Design review of the part built by this model. Coordinates are the model's own, in mm. Face numbers are marked on the shaded views. A direction names the side the tool comes from. Coordinates: 2 decimals unless noted, no trailing zeros. Write each loop counter-clockwise with the first axis right and the second up, starting at its lowest first coordinate (ties: lowest second). Pieces come first, ordered by that corner, then holes. Notation, with made-up numbers: (-13, 63) - (42, 63) arc R17 cw to (42, 81) - close; hole circle Ø11 at (76.5, 46). An arc over 180 degrees is marked (long way). One line per item, written item: value.
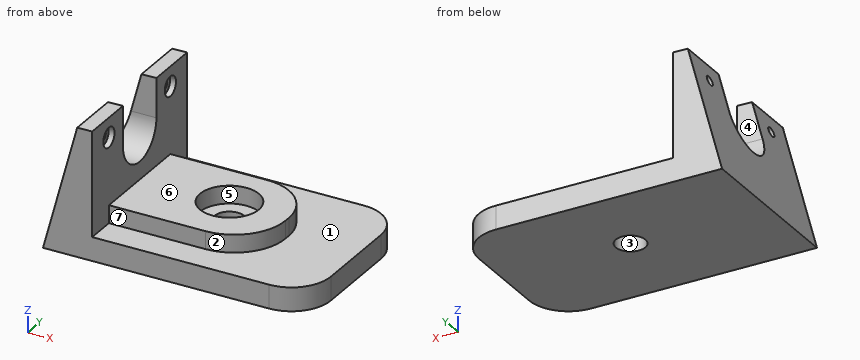
Autodesk Fusion 360 part; units mm, degrees
sketch "Baza" plane through (0, 0, 0) normal (0, 0, 1) x (1, 0, 0)
  line L0 (0, 0) -> (0, 85)
  line L1 (0, 85) -> (135, 85)
  line L2 (135, 85) -> (135, 0)
  line L3 (135, 0) -> (0, 0)
  line L4 (0, 0) -> (25, 0) construction
  line L5 (25, 0) -> (25, 85)
  line L6 (25, 85) -> (25, 70) construction
  line L7 (25, 0) -> (25, 15) construction
  line L8 (69.701, 85) -> (69.701, 0) construction
  line L9 (135, 85) -> (69.701, 44.195) construction
  circle A0 centre (69.701, 44.195) radius 7.5
  circle A1 centre (69.701, 44.195) radius 15
  line L10 (25, 70) -> (100, 70)
  line L11 (100, 70) -> (100, 15)
  line L12 (100, 15) -> (25, 15)
  line L13 (25, 15) -> (25, 70)
  dimension "d1" = 85
  dimension "d2" = 135
  dimension "d3" = 25
  dimension "d4" = 15
  dimension "d5" = 15
  dimension "d6" = 77
  dimension "d7" = 15
  dimension "d8" = 30
  dimension "d9" = 55
  dimension "d10" = 44.701
  dimension "d11" = 35
extrude "Extrude1" add sketch "Baza" along normal blind 12 contours L0 L1 L3 L5 L13 | L1 L2 L3 L5 L10 L11 L12 | L5 L10 L11 L12 L13 | A0 | A1 makes body 1
extrude "Extrude2" add sketch "Baza" along normal blind 21 separate body contours L5 L10 L11 L12 L13 makes body 2
combine "Combine1" operation add target body 2 tool bodies 1
extrude "Extrude3" cut sketch "Baza" along normal blind 50 contours A0 bodies 2
fillet "Fillet1" radius 26 2 edges at (100, 15, 16.5) (100, 70, 16.5) on bodies 2
fillet "Fillet2" radius 20 2 edges at (135, 0, 6) (135, 85, 6) on bodies 2
sketch "Margine" plane through (0, 0, 0) normal (0, -1, 0) x (1, 0, 0)
  line L0 (115, 0) -> (115, 12)
  line L1 (115, 12) -> (0, 12)
  line L2 (0, 12) -> (0, 0)
  line L3 (0, 0) -> (115, 0)
  line L4 (0, 0) -> (25, 0) construction
  line L5 (25, 0) -> (25, 65)
  line L6 (0, 0) -> (17.3848, 64.881)
  line L7 (0, 0) -> (67.1698, 0) construction
  line L8 (17.3848, 64.881) -> (25, 65)
  line L9 (3.2154, 12) -> (25, 12)
  line L10 (3.2154, 12) -> (0, 12)
  line L11 (0, 0) -> (0, 12)
  dimension "d22" = 25
  dimension "d23" = 65
  dimension "d24" = 75
extrude "Extrude4" add sketch "Margine" against normal blind 85 contours L1 L5 L6 L8 L9 bodies 2
extrude "Extrude5" cut sketch "Margine" against normal blind 85 contours L1 L2 L6 L10 L11 bodies 2
sketch "Fata" plane through (25, 0, 0) normal (1, 0, 0) x (0, 1, 0)
  line L0 (70, 21) -> (70, 12)
  line L1 (70, 12) -> (85, 12)
  line L2 (85, 12) -> (85, 65)
  line L3 (85, 65) -> (0, 65)
  line L4 (0, 65) -> (0, 12)
  line L5 (0, 12) -> (15, 12)
  line L6 (15, 12) -> (15, 21)
  line L7 (15, 21) -> (70, 21)
  line L8 (0, 65) -> (15, 65) construction
  line L9 (85, 65) -> (70, 65) construction
  line L10 (15, 65) -> (15, 55) construction
  line L11 (70, 65) -> (70, 55) construction
  circle A0 centre (15, 55) radius 2.5
  circle A1 centre (70, 55) radius 2.5
  circle A2 centre (15, 55) radius 5
  circle A3 centre (70, 55) radius 5
  line L12 (0, 65) -> (0, 45) construction
  line L13 (0, 45) -> (85, 45) construction
  line L14 (27.5, 45) -> (27.5, 65)
  line L15 (57.5, 45) -> (57.5, 65)
  arc A4 (27.5, 45) -> (57.5, 45) centre (42.5, 45) ccw
  dimension "d29" = 15
  dimension "d30" = 15
  dimension "d31" = 10
  dimension "d32" = 10
  dimension "d33" = 5
  dimension "d34" = 5
  dimension "d35" = 10
  dimension "d36" = 10
  dimension "d37" = 20
  dimension "d40" = 30
extrude "Extrude6" cut sketch "Fata" against normal blind 20 contours L3 L14 L15 A4 bodies 2
extrude "Extrude7" cut sketch "Fata" against normal blind 15 contours A0 | A1 bodies 2
extrude "Extrude8" cut sketch "Fata" against normal blind 3 contours A2 | A3 bodies 2
1. Mouldability with a two-part tool opening along X and no side actions: class the marked faces 1, 2 and 3 as released by +X, released by -X, zero draft, split by the parting line, or undercut.
Answer block:
face 1: zero draft
face 2: released by +X
face 3: undercut
2. Wall thickness on line 1 along Y through (x, z) = (16.5, 55); line 2 along Y through (x, z) = (24, 62); line 3 along Z through (x, y) = (18.25, 70): over which ranges is each line inside the solid? List them lowest first.
Answer block:
line 1: y = 0 to 12.5, 17.5 to 27.5, 57.5 to 67.5, 72.5 to 85
line 2: y = 0 to 27.5, 57.5 to 85
line 3: z = 0 to 52.5, 57.5 to 64.89
3. Insertion check: pin 1 Ø1.5 at (x, z) = (15, 13) entering from -Y; pin 2 Ø3 at (y, z) = (68, 53.5) entering from +X; pin 3 Ø3 at (x, y) = (61, 39) entering from +Z; pin 4 Ø4.5 at (x, z) = (53, 16.5) entering from -Y. Each pin has a flat end and moves straight along its axis. Give the tip position at first contact, or say it passes through.
Answer block:
pin 1: stops at y = 0
pin 2: stops at x = 22
pin 3: stops at z = 12
pin 4: stops at y = 15
4. Consider section D-D, the plane x = 70. Write out the cut boundary in (y, z), then the cut area to 3 significant figures.
Answer block:
outline: (0, 0) - (36.7, 0) - (36.7, 12) - (29.2, 12) - (29.2, 21) - (15, 21) - (15, 12) - (0, 12) - close; (51.69, 0) - (85, 0) - (85, 12) - (70, 12) - (70, 21) - (59.19, 21) - (59.19, 12) - (51.69, 12) - close
area: 1,070 mm^2
5. For the marked faces 4, 5, 6 and 7, list the 3-axis set-ups (+Z, -Z, +X, -X, +Y, -Y) from which the entire face can be reached by the end or side of a thin tool; tool diameter is ignored.
Answer block:
face 4: +Z, +X, -X
face 5: +Z
face 6: +Z, +X, +Y, -Y
face 7: +Z, +X, -Y
6. Consider section A-A, the plane x = 98. Write out the cut boundary in (y, z), then the cut area to 3 significant figures.
Answer block:
outline: (0, 0) - (85, 0) - (85, 12) - (54, 12) - (54, 21) - (31, 21) - (31, 12) - (0, 12) - close
area: 1,230 mm^2
7. Consider section B-B, the plane y = 42.5. Write out the cut boundary in (x, z), then the cut area to 3 significant figures.
Answer block:
outline: (0, 0) - (62.4, 0) - (62.4, 12) - (54.8, 12) - (54.8, 21) - (25, 21) - (25, 30) - (8.04, 30) - close; (77.01, 0) - (135, 0) - (135, 12) - (100, 12) - (100, 21) - (84.6, 21) - (84.6, 12) - (77.01, 12) - close
area: 2,180 mm^2
8. Consider section C-C, the plane z = 15. Write out the cut boundary in (x, y) (3 decimals), then the cut area to 3 significant figures.
Answer block:
outline: (4.019, 0) - (25, 0) - (25, 15) - (74, 15) arc R26 ccw to (100, 41) - (100, 44) arc R26 ccw to (74, 70) - (25, 70) - (25, 85) - (4.019, 85) - close; hole circle Ø30 at (69.701, 44.195)
area: 4,910 mm^2
